Can you work these out from the model? Positions are in its coordinate system, mm. A direction names the side the tool comes from. Round coordinates to 2 decimals unless told otherwise and drop trailing zeros. Loops run counter-clockwise (first coordinate to the right, second up) from the corner with the lowest first, then second, coordinate; pieces in that order, holes last.
(1) Which directions (+Z, -Z, +X, -X, +Y, -Y) give clear straight access to the entire face, cutting with the end or side of a thin tool? Please do faces 1 (the face through (-4, 5, 65)), 2 (the face through (0, 8, 45)), 3 (the face through (4, 5, -65)), 4 (the face through (0, 11, 60)).
(2) I want a section at C-C on x = -12.25. Write out the boundary of the cut face in (y, z).
(3) I want a section at B-B on x = 0. Write out the boundary of the cut face in (y, z), plus the area to 3 significant figures.
(4) I want a section at D-D on z = -37.5. Write out the boundary of the cut face in (x, y).
(5) If I drill on line 1 along Z through (x, y) = (0, 1.25); line 2 along Z through (x, y) = (0, 6.35); line 3 along Z through (x, y) = (-10, 7.5), over which ranges is the centre line in solid material (lowest first)?
(6) Will these pins go through, and if not, where does the flat tip stop? pin 1 Ø3 at (x, z) = (7, -32.5) entering from +Y; pin 2 Ø1 at (x, y) = (0, 3) entering from -Z; pin 3 Ø10 at (x, z) = (0, 65) entering from -Y.
(7) I want a section at A-A on z = -65. Write out the boundary of the cut face in (x, y).
(8) Thinking about a two-plate mould opening in Z: for faces 5 (the face through (-0.267, 2.535, -39.533)), 6 (the face through (0, 3, 55)), 7 (the face through (0, 8, -75)), 8 (the face through (15, 4, -1)), which applies, released by +Z, released by -Z, zero draft, split by the parting line, or undercut?
Autodesk Inventor part; units mm, degrees
ref_plane "YZ Plane" through (0, 0, 0) normal (1, 0, 0) x (0, 1, 0)
ref_plane "XZ Plane" through (0, 0, 0) normal (0, 1, 0) x (-1, 0, 0)
ref_plane "XY Plane" through (0, 0, 0) normal (0, 0, 1) x (1, 0, 0)
sketch "Skizze1" plane through (0, 0, 0) normal (0, 1, 0) x (-1, 0, 0)
  line L0 (-15, 50) -> (15, 50)
  line L1 (15, 50) -> (15, -50)
  line L2 (15, -50) -> (-15, -50)
  line L3 (-15, -50) -> (-15, 50)
  line L4 (-15, 50) -> (15, -50) construction
  line L5 (15, 50) -> (-15, -50) construction
  point P0 (0, 0)
  dimension "d0" = 30
  dimension "d1" = 100
extrude "Extrusion1" add sketch "Skizze1" along normal blind 5
sketch "Skizze2" plane through (0, 5, 0) normal (0, 1, 0) x (1, 0, 0)
  line L0 (15, 50) -> (-15, 50)
  line L1 (-15, 50) -> (-15, -50)
  line L2 (-15, -50) -> (15, -50)
  line L3 (15, -50) -> (15, 50)
  line L4 (-15, -50) -> (15, -50)
  line L5 (0, -37.5) -> (0, 37.5)
  circle A0 centre (0, -37.5) radius 2.05
  circle A1 centre (0, 37.5) radius 2.05
  point P0 (0, 0)
  dimension "d22" = 75
  dimension "d23" = 4.1
  dimension "d24" = 4.1
sketch "Skizze3" plane through (0, 5, 0) normal (0, 1, 0) x (1, 0, 0)
  line L0 (-15, -50) -> (15, -50)
  line L1 (-15, -50) -> (0, -50)
  line L2 (0, -37.5) -> (0, 37.5)
  circle A0 centre (0, -37.5) radius 2.05
  circle A1 centre (0, 37.5) radius 2.05
  line L3 (15, -50) -> (15, 50)
  line L4 (-15, -50) -> (15, -50)
  line L5 (15, -50) -> (15, -45)
  line L6 (15, -45) -> (-15, -45)
  line L7 (-15, -45) -> (-15, -50)
  line L8 (-15, 50) -> (15, 50)
  line L9 (15, 50) -> (15, 45)
  line L10 (15, 45) -> (-15, 45)
  line L11 (-15, 45) -> (-15, 50)
  point P0 (0, 0)
  dimension "d4" = 15
  dimension "d5" = 12.5
  dimension "d6" = 75
  dimension "d7" = 4.1
  dimension "d8" = 4.1
  dimension "d9" = 5
  dimension "d10" = 5
extrude "Extrusion2" add sketch "Skizze3" along normal blind 6 contours L7 L6 L3 L0 | L10 L11 L8 L3
sketch "Skizze4" plane through (-15, 0, 50) normal (0, 0, 1) x (1, 0, 0)
  line L0 (0, 0) -> (30, 0)
  line L1 (30, 0) -> (30, 11)
  line L2 (0, 11) -> (30, 11)
  line L3 (0, 0) -> (0, 11)
  line L4 (0, 5) -> (30, 5)
  point P0 (15, 0)
extrude "Extrusion3" add sketch "Skizze4" along normal blind 25 contours L3 L2 L1 L4
sketch "Skizze5" plane through (15, 0, -50) normal (0, 0, -1) x (-1, 0, 0)
  line L0 (0, 0) -> (30, 0)
  line L1 (30, 0) -> (30, 11)
  line L2 (0, 11) -> (30, 11)
  line L3 (0, 0) -> (0, 11)
  line L4 (0, 5) -> (30, 5)
  point P0 (15, 0)
extrude "Extrusion4" add sketch "Skizze5" along normal blind 25 contours L3 L2 L1 L4
sketch "Skizze6" plane through (15, 0, -50) normal (0, 0, -1) x (-1, 0, 0)
  line L0 (0, 5) -> (30, 5)
  line L1 (0, 0) -> (30, 0)
  line L2 (30, 5) -> (0, 5)
  line L3 (0, 0) -> (0, 5)
  line L4 (0, 0) -> (30, 0)
  line L5 (30, 0) -> (30, 5)
  point P0 (15, 0)
extrude "Extrusion5" add sketch "Skizze6" along normal blind 5
sketch "Skizze7" plane through (-15, 0, 50) normal (0, 0, 1) x (1, 0, 0)
  line L0 (30, 5) -> (0, 5)
  line L1 (0, 0) -> (0, 5)
  line L2 (0, 0) -> (30, 0)
  line L3 (30, 0) -> (30, 5)
  point P0 (15, 0)
extrude "Extrusion6" add sketch "Skizze7" along normal blind 5
extrude "Extrusion7" cut sketch "Skizze2" against normal blind 5 contours A1 | A0
sketch "Skizze8" plane through (0, 11, 0) normal (0, 1, 0) x (1, 0, 0)
  line L0 (15, -45) -> (15, -75)
  line L1 (15, -45) -> (-15, -45)
  line L2 (-15, -45) -> (-15, -75)
  line L3 (15, -75) -> (-15, -75)
  line L4 (0, -75) -> (0, -65)
  circle A0 centre (0, -65) radius 3.1
  line L5 (-15, 45) -> (-15, 75)
  line L6 (-15, 45) -> (15, 45)
  line L7 (15, 45) -> (15, 75)
  line L8 (-15, 75) -> (15, 75)
  line L9 (0, 75) -> (0, 65)
  circle A1 centre (0, 65) radius 3.1
  point P0 (0, 0)
  dimension "d27" = 10
  dimension "d28" = 6.2
  dimension "d29" = 10
  dimension "d30" = 6.2
extrude "Extrusion8" cut sketch "Skizze8" against normal blind 7 contours A0 | A1
properties part number "DepthCAM"
Filled sheet:
1. face 1: +Z, +X, -X, -Y
1. face 2: +X, -X, +Y
1. face 3: -Z, +X, -X, -Y
1. face 4: +Z, -Z, +X, -X, +Y
2. outline: (0, -55) - (5, -55) - (5, -75) - (11, -75) - (11, -45) - (5, -45) - (5, 45) - (11, 45) - (11, 75) - (5, 75) - (5, 55) - (0, 55) - close
3. outline: (0, -55) - (5, -55) - (5, -61.9) - (11, -61.9) - (11, -45) - (5, -45) - (5, -39.55) - (0, -39.55) - close; (0, -35.45) - (5, -35.45) - (5, 35.45) - (0, 35.45) - close; (0, 39.55) - (5, 39.55) - (5, 45) - (11, 45) - (11, 61.9) - (5, 61.9) - (5, 55) - (0, 55) - close; (5, -75) - (11, -75) - (11, -68.1) - (5, -68.1) - close; (5, 68.1) - (11, 68.1) - (11, 75) - (5, 75) - close
3. area: 795 mm2
4. outline: (-15, 0) - (-2.05, 0) - (-2.05, 5) - (-15, 5) - close; (2.05, 0) - (15, 0) - (15, 5) - (2.05, 5) - close
5. line 1: z = -55 to -39.55, -35.45 to 35.45, 39.55 to 55
5. line 2: z = -75 to -68.1, -61.9 to -45, 45 to 61.9, 68.1 to 75
5. line 3: z = -75 to -45, 45 to 75
6. pin 1: stops at y = 5
6. pin 2: stops at z = -55
6. pin 3: stops at y = 5
7. outline: (-15, 5) - (-3.1, 5) - (-3.1, 11) - (-15, 11) - close; (3.1, 5) - (15, 5) - (15, 11) - (3.1, 11) - close
8. face 5: undercut
8. face 6: released by +Z
8. face 7: released by -Z
8. face 8: zero draft
